Source: CAD feature listing. Evaluate the final solid. Frame: model axes, mm. A direction names the side the tool comes from. Coordinates: 2 decimals unless noted, no trailing zeros. Order: outer loops, then holes, each group sorted by start corner. A loop starts at its lowest first (then second) coordinate and runs counter-clockwise, first axis right, second up. Notation, with made-up numbers: (-8.5, -23.75) - (25.5, -23.75) arc R30 cw to (25.5, 3.25) - close; hole circle Ø4 at (58.5, -14). An arc over 180 degrees is marked (long way). One line per question, with ' | ' between items. Start each with the question number.
(1) Contact query for flat-ended pins moving along their axis: P1, Ø10, axis at x = -33.5, y = 15, coming from the -Z side; P2, Ø12, axis at x = 38, y = 16, coming from the -Z side; P3, Ø1.5, axis at y = 42.5, z = 26.5, coming from the +X side. Output: stop coordinate, or through.
(2) Draft query along Z for faces 3 (the cylindrical face through (-45.783, 20.28, -14.418)), 4 (the flat face through (21, 0, 10)), 5 (the flat face through (-16.4, 7, 16.4)). Return one class per face: +Z half, -Z half, draft (parallel to the pull), parting line (faces both ways), or undercut.
(3) Line query: line 1 along Z through (x, y) = (0, 23); line 2 along Z through (x, y) = (0, 5.5); line 3 along Y through (x, z) = (-28, 13.5). Output: solid intervals per line, ascending.
(4) Section C-C (y = 20.5). Return the cut outline in (x, z), then the cut area to 3 significant figures.
(5) Access query for faces 1 (the cylindrical face through (8.238, 28.199, 37.096)), 2 (the cylindrical face through (10.382, 3.549, -19.961)). Directions: +Z, -Z, +X, -X, +Y, -Y. A direction counts if a zero-diameter tool reaches every point of the face in a straight line with its end or side. Return the directions, or none.
from build123d import *

# Parameters (mm, degrees)
CUT_EXTRUDE1_DEPTH      = 85.308955633
CUT_EXTRUDE1_DEPTH_BACK = 85.308955633
SKETCH2_R               = 22.5
CHAMFER1_SIZE           = 10


with BuildPart() as part:
    # Sketch1 → Revolve2 (revolve)
    with BuildSketch(Plane.XY, mode=Mode.PRIVATE) as revolve2_sk:
        Polygon((0, 0), (48, 0), (48, 50), (38, 50), (38, 7), (0, 7), align=None)
    revolve(revolve2_sk.sketch.rotate(Axis((0, 7, 0), (0, -1, 0)), 180), axis=Axis((0, 7, 0), (0, -1, 0)))

    # Sketch2 → Cut-Extrude1 (cut, two sides: drawn at the far end of the back side and taken through both)
    with BuildSketch(Plane.XZ.offset(-CUT_EXTRUDE1_DEPTH_BACK)):
        Circle(SKETCH2_R)
    extrude(amount=CUT_EXTRUDE1_DEPTH + CUT_EXTRUDE1_DEPTH_BACK, mode=Mode.SUBTRACT)

    # Chamfer1
    chamfer1_edges = [part.edges().sort_by_distance(p)[0] for p in [
        (48, 50, 0),
    ]]
    chamfer(chamfer1_edges, length=CHAMFER1_SIZE - 0.0001)  # a hair under: the kernel refuses the full size


solid = part.part
Response values:
1) P1: stops at z = -38.62 | P2: stops at z = -35.78 | P3: stops at x = 38.04
2) face 3: parting line | face 4: draft | face 5: undercut
3) line 1: z = -48 to -38, 38 to 48 | line 2: z = -48 to -22.5, 22.5 to 48 | line 3: y = 0 to 7
4) outline: circle Ø96 at (0, 0); hole circle Ø76 at (0, 0) | area: 2,700 mm²
5) face 1: +Y | face 2: +Y, -Y
